Read the model definition and answer for the solid it produces. Units are mm, in the model's axes. A direction names the side the tool comes from. Coordinates: 2 decimals unless noted, no trailing zeros. Loops run counter-clockwise (first coordinate to the right, second up) from the corner with the lowest first, then second, coordinate; pieces in that order, holes last.
from build123d import *

# Parameters (mm, degrees)
BOSS_EXTRUDE1_DEPTH = 8
CUT_EXTRUDE1_DEPTH  = 38.332956939


with BuildPart() as part:
    # Sketch1 → Boss-Extrude1 (new body)
    with BuildSketch(Plane.YZ):
        with BuildLine():
            Line((21.778218983, -15.260770999), (22.403447361, -16.090477082))
            ThreePointArc((22.403447361, -16.090477082), (21.256795907, -17.969098146), (21.458282303, -20.160770999))
            Line((21.458282303, -20.160770999), (-7.771266811, -20.160770999))
            ThreePointArc((-7.771266811, -20.160770999), (-9.271266811, -21.660770999), (-7.771266811, -23.160770999))
            Line((-7.771266811, -23.160770999), (26.228733189, -23.160770999))
            Line((26.228733189, -23.160770999), (25.478499604, -22.165177406))
            ThreePointArc((25.478499604, -22.165177406), (28.142104739, -18.351761478), (24.66608529, -15.260770999))
            Line((24.66608529, -15.260770999), (21.778218983, -15.260770999))
        make_face()
    extrude(amount=BOSS_EXTRUDE1_DEPTH)

    # Sketch2 → Cut-Extrude1 (cut, through all)
    with BuildSketch(Plane(origin=(0, 0, 0), x_dir=(0, -1, 0), z_dir=(-1, 0, 0))):
        with BuildLine():
            ThreePointArc((-22.283084357, -15.93074998), (-22.602512003, -16.109797243), (-22.254615534, -16.224077557))
            ThreePointArc((-22.254615534, -16.224077557), (-22.328076964, -16.156214018), (-22.403447361, -16.090477082))
            Line((-22.403447361, -16.090477082), (-22.283084357, -15.93074998))
        make_face()
        with BuildLine():
            ThreePointArc((-21.458282303, -20.160770999), (-21.383523815, -19.975180388), (-21.319492659, -19.785621116))
            ThreePointArc((-21.319492659, -19.785621116), (-21.83451901, -20.296586831), (-21.111872142, -20.360770999))
            Line((-21.111872142, -20.360770999), (-21.458282303, -20.160770999))
        make_face()
        with BuildLine():
            Line((-25.478499604, -22.165177406), (-25.598862609, -22.324904508))
            ThreePointArc((-25.598862609, -22.324904508), (-25.289362351, -22.100161258), (-25.671631303, -22.113214469))
            ThreePointArc((-25.671631303, -22.113214469), (-25.575436693, -22.140575731), (-25.478499604, -22.165177406))
        make_face()
        with BuildLine():
            ThreePointArc((7.771266811, -20.160770999), (7.383968477, -20.211633325), (7.022935334, -20.360770999))
            Line((7.022935334, -20.360770999), (-21.111872142, -20.360770999))
            Line((-21.111872142, -20.360770999), (-21.458282303, -20.160770999))
            Line((-21.458282303, -20.160770999), (7.771266811, -20.160770999))
        make_face()
        with BuildLine():
            Line((-21.319492659, -20.160770999), (-21.319492659, -19.785621116))
            ThreePointArc((-21.319492659, -19.785621116), (-21.383523815, -19.975180388), (-21.458282303, -20.160770999))
            Line((-21.458282303, -20.160770999), (-21.319492659, -20.160770999))
        make_face()
        with BuildLine():
            Line((-25.671631303, -22.113214469), (-25.598862609, -22.324904508))
            Line((-25.598862609, -22.324904508), (-25.478499604, -22.165177406))
            ThreePointArc((-25.478499604, -22.165177406), (-25.575436693, -22.140575731), (-25.671631303, -22.113214469))
        make_face()
        with BuildLine():
            ThreePointArc((-22.403447361, -16.090477082), (-22.328076964, -16.156214018), (-22.254615534, -16.224077557))
            Line((-22.254615534, -16.224077557), (-22.283084357, -15.93074998))
            Line((-22.283084357, -15.93074998), (-22.403447361, -16.090477082))
        make_face()
    extrude(amount=-CUT_EXTRUDE1_DEPTH, mode=Mode.SUBTRACT)


solid = part.part
Item 1: Determine the mould class of faces 1 (the face through (4, 9, -23.161)), 2 (the face through (3.9, 21.3, -17.8)), 3 (the face through (4, 7, -20.361)) for opening direction Z: released by +Z, released by -Z, zero draft, split by the parting line, or undercut.
Numbers:
face 1: released by -Z
face 2: undercut
face 3: released by +Z
Item 2: A cutting plane is placed at A-A on y = -1. Determine the outline of the cut face in (x, z).
Numbers:
outline: (0, -23.16) - (8, -23.16) - (8, -20.36) - (0, -20.36) - close
Item 3: Which of the six approach directions +Z, -Z, +X, -X, +Y, -Y give full straight-line access (tool end or side, diameter ignored) to faces 4 (the face through (4, 23, -15.261)), 5 (the face through (3.94, 25.92, -22.75))?
Numbers:
face 4: +Z, +X, -X, +Y, -Y
face 5: +X, -X, +Y
Item 4: A cutting plane is placed at C-C on z = -21.25. Determine the outline of the cut face in (x, y).
Numbers:
outline: (0, -9.21) - (8, -9.21) - (8, 27.13) - (0, 27.13) - close
Item 5: A cutting plane is placed at B-B on x = 7. Determine the outline of the cut face in (y, z).
Numbers:
outline: (-7.77, -23.16) - (26.23, -23.16) - (25.6, -22.32) arc R0.2 cw (long way) to (25.67, -22.11) arc R3.5 ccw to (24.67, -15.26) - (21.78, -15.26) - (22.28, -15.93) arc R0.2 cw (long way) to (22.25, -16.22) arc R3.5 ccw to (21.32, -19.79) arc R0.4 cw (long way) to (21.11, -20.36) - (-7.02, -20.36) arc R1.5 ccw (long way) to start
Item 6: Find the intervals of material crossed by line 1 along Y through (x, z) = (6.25, -19); line 2 along Z through (x, y) = (7, -2.5); line 3 along Z through (x, y) = (5.5, 22.5), in increasing order.
Numbers:
line 1: y = 21.17 to 28.16
line 2: z = -23.16 to -20.36
line 3: z = -23.16 to -16.27, -15.92 to -15.26
Item 7: Given pin 1 (2 mm diameter, centred on x = 1, y = -0.5, fed in from +Z); pin 2 (1 mm diameter, centred on x = 5.5, z = -16.5, fed in from -Y), each flat-ended and moving along its own axis, determine where each tip first touches the part or whether it passes through.
Numbers:
pin 1: stops at z = -20.36
pin 2: stops at y = 21.64
